Read the model definition and answer for the solid it produces. Units are mm, in the model's axes. A direction names the side the tool comes from. Coordinates: 2 decimals unless noted, no trailing zeros. Order: outer loops, then holes, each group sorted by start corner. A loop starts at its lowest first (then second) coordinate and runs counter-clockwise, first axis right, second up. Notation, with made-up numbers: (-19, 33) - (-9, 33) arc R24 cw to (-9, 59) - close; hole circle Ø2 at (-18.5, 17). An arc over 180 degrees is marked (long way). Use one line per item in the form item = value.
```python
from build123d import *

# Parameters (mm, degrees)
BOSS_EXTRUDE1_DEPTH     = 1.5875
F_1_4_CLEARANCE_HOLE1_D = 7.14248


with BuildPart() as part:
    # Sketch1 → Boss-Extrude1 (new, symmetric)
    with BuildSketch(Plane(origin=(0, 0, 0), x_dir=(1, 0, 0), z_dir=(0, 1, 0))):
        Polygon((-108.508102479, 122.649104887), (-99.990490133, 132.8), (99.990490133, 132.8), (108.508102479, 122.649104887), (126.560486405, 125.832227239), (132.451914797, 118.811096288), (126.182387654, 101.585712032), (134.7, 91.434816919), (134.7, -91.434816919), (126.182387654, -101.585712032), (132.451914797, -118.811096288), (126.560486405, -125.832227239), (108.508102479, -122.649104887), (99.990490133, -132.8), (-99.990490133, -132.8), (-108.508102479, -122.649104887), (-126.560486405, -125.832227239), (-132.451914797, -118.811096288), (-126.182387654, -101.585712032), (-134.7, -91.434816919), (-134.7, 91.434816919), (-126.182387654, 101.585712032), (-132.451914797, 118.811096288), (-126.560486405, 125.832227239), align=None)
        Polygon((-95.327413552, 122.8), (-124.7, 87.795114576), (-124.7, 49.5), (-117.031174581, 49.5), (-117.031174581, 34.92759842), (-124.7, 30.5), (-124.7, -30.5), (-117.031174581, -34.92759842), (-117.031174581, -49.5), (-124.7, -49.5), (-124.7, -87.795114576), (-95.327413552, -122.8), (-87, -122.8), (-87, -115.131174581), (-83.825, -115.131174581), (-79.39740158, -122.8), (-7.681406121, -122.8), (-4.274808593, -116.8996), (4.274808593, -116.8996), (7.681406121, -122.8), (79.39740158, -122.8), (83.825, -115.131174581), (87, -115.131174581), (87, -122.8), (95.327413552, -122.8), (124.7, -87.795114576), (124.7, -49.5), (117.031174581, -49.5), (117.031174581, -34.92759842), (124.7, -30.5), (124.7, 30.5), (117.031174581, 34.92759842), (117.031174581, 49.5), (124.7, 49.5), (124.7, 87.795114576), (95.327413552, 122.8), (87, 122.8), (87, 115.131174581), (83.825, 115.131174581), (79.39740158, 122.8), (7.681406121, 122.8), (4.274808593, 116.8996), (-4.274808593, 116.8996), (-7.681406121, 122.8), (-79.39740158, 122.8), (-83.825, 115.131174581), (-87, 115.131174581), (-87, 122.8), align=None, mode=Mode.SUBTRACT)
    extrude(amount=BOSS_EXTRUDE1_DEPTH, both=True)

    # 1/4 Clearance Hole1 (through all)
    with Locations(Plane(origin=(0, -1.5875, 0), x_dir=(-1, 0, 0), z_dir=(0, -1, 0))):
        with Locations((-123.415994069, 117.211371709), (-126.7498, 40), (0, 124.8498), (123.415994069, 117.211371709), (126.7498, 40), (126.7498, -40), (123.415994069, -117.211371709), (0, -124.8498), (-123.415994069, -117.211371709), (-126.7498, -40)):
            Hole(F_1_4_CLEARANCE_HOLE1_D / 2)


solid = part.part
```
(1) Section B-B, the plane z = -40 is taken. Write down the section's boundary in (x, y).
Answer list:
outline = (-134.7, -1.59) - (-130.32, -1.59) - (-130.32, 1.59) - (-134.7, 1.59) - close; (-123.18, -1.59) - (-117.03, -1.59) - (-117.03, 1.59) - (-123.18, 1.59) - close; (117.03, -1.59) - (123.18, -1.59) - (123.18, 1.59) - (117.03, 1.59) - close; (130.32, -1.59) - (134.7, -1.59) - (134.7, 1.59) - (130.32, 1.59) - close
(2) Section A-A, the plane x = 0 is taken. Write down the section's boundary in (y, z).
Answer list:
outline = (-1.59, -132.8) - (1.59, -132.8) - (1.59, -128.42) - (-1.59, -128.42) - close; (-1.59, -121.28) - (1.59, -121.28) - (1.59, -116.9) - (-1.59, -116.9) - close; (-1.59, 116.9) - (1.59, 116.9) - (1.59, 121.28) - (-1.59, 121.28) - close; (-1.59, 128.42) - (1.59, 128.42) - (1.59, 132.8) - (-1.59, 132.8) - close
(3) The mould has two halves that part along Z. Classify faces 1 (the flat face through (0.6, -1.588, 117.4)), 2 (the flat face through (110.22, 0.02, -105.05)), 3 (the flat face through (129.465, 0.022, -122.371)): +Z half, -Z half, draft (parallel to the pull), parting line (faces both ways), or undercut.
Answer list:
face_1 = draft
face_2 = undercut
face_3 = -Z half
(4) Which of the six approach directions +Z, -Z, +X, -X, +Y, -Y give full straight-line access (tool end or side, diameter ignored) to faces 4 (the flat face through (-110.22, 0.02, 105.05)), 5 (the flat face through (-104.31, 0.02, -127.65)), 6 (the flat face through (-129.36, 0.02, 110.32)), 7 (the flat face through (130.5, 0.02, 96.44))?
Answer list:
face_4 = +Y, -Y
face_5 = -Z, +Y, -Y
face_6 = -X, +Y, -Y
face_7 = +X, +Y, -Y
(5) Given pin 1 Ø1 at (x, y) = (122, 0) entering from +Z; pin 2 Ø1 at (y, z) = (0.5, 119) entering from +X, each flat-ended and moving along its own axis, determine where each tip first touches the part or whether it passes through.
Answer list:
pin_1 = 125.12
pin_2 = 132.45
(6) Section C-C, the plane x = 58 is taken. Write down the section's boundary in (y, z).
Answer list:
outline = (-1.59, -132.8) - (1.59, -132.8) - (1.59, -122.8) - (-1.59, -122.8) - close; (-1.59, 122.8) - (1.59, 122.8) - (1.59, 132.8) - (-1.59, 132.8) - close
(7) Section D-D, the plane z = 22 is taken. Write down the section's boundary in (x, y).
Answer list:
outline = (-134.7, -1.59) - (-124.7, -1.59) - (-124.7, 1.59) - (-134.7, 1.59) - close; (124.7, -1.59) - (134.7, -1.59) - (134.7, 1.59) - (124.7, 1.59) - close
(8) Straight lines are drawn through the part: L1, parallel to Z at x = 55, y = -1.1; L2, parallel to X at y = 0.7, z = -40; L3, parallel to X at y = 1.2, z = -22.5. For each, find the intervals that lie inside material, in ascending order.
Answer list:
L1 = -132.8 to -122.8, 122.8 to 132.8
L2 = -134.7 to -130.32, -123.18 to -117.03, 117.03 to 123.18, 130.32 to 134.7
L3 = -134.7 to -124.7, 124.7 to 134.7
